Could you check a few things on this model? Use its own coordinates, in mm. Face numbers are marked on the shaded views. A direction names the side the tool comes from. Coordinates: 2 decimals unless noted, no trailing zeros. Loops run counter-clockwise (first coordinate to the right, second up) from the corner with the lowest first, then second, coordinate; pieces in that order, holes last. Notation, with made-up numbers: (5, 73) - (19, 73) arc R23 cw to (19, 99) - close; hole circle Ø5 at (-12.75, 46). An arc over 180 degrees is marked (long way). Put each result on its own line as item: value. Start each with the question number.
```python
from build123d import *

# Parameters (mm, degrees)
F0_R     = 3.175
F1_DEPTH = 12.7


with BuildPart() as f1:
    # F0 (on Front) → F1 (new body)
    with BuildSketch(Plane.XZ):
        with BuildLine():
            Line((0.507003, 7.684488), (0.507003, 6.329727))
            ThreePointArc((0.507003, 6.329727), (0, 6.35), (-0.507003, 6.329727))
            Line((-0.507003, 6.329727), (-0.507003, 7.684488))
            Line((-0.507003, 7.684488), (-0.257541, 7.684488))
            Line((-0.257541, 7.684488), (-0.257541, 7.937779))
            Line((-0.257541, 7.937779), (-0.507003, 7.937779))
            Line((-0.507003, 7.937779), (-1.277548, 7.937779))
            Line((-1.277548, 7.937779), (-1.277548, 6.220158))
            ThreePointArc((-1.277548, 6.220158), (-5.499261, 3.175), (-6.025589, -2.00369))
            Line((-6.025589, -2.00369), (-7.513093, -2.8625))
            Line((-7.513093, -2.8625), (-7.12782, -3.529812))
            Line((-7.12782, -3.529812), (-7.003089, -3.745852))
            Line((-7.003089, -3.745852), (-6.783733, -3.619207))
            Line((-6.783733, -3.619207), (-6.908463, -3.403167))
            Line((-6.908463, -3.403167), (-5.735206, -2.725786))
            ThreePointArc((-5.735206, -2.725786), (-5.499261, -3.175), (-5.228203, -3.603941))
            Line((-5.228203, -3.603941), (-6.401461, -4.281321))
            Line((-6.401461, -4.281321), (-6.526191, -4.065281))
            Line((-6.526191, -4.065281), (-6.745548, -4.191927))
            Line((-6.745548, -4.191927), (-6.620817, -4.407967))
            Line((-6.620817, -4.407967), (-6.235544, -5.075279))
            Line((-6.235544, -5.075279), (-4.748041, -4.216469))
            ThreePointArc((-4.748041, -4.216469), (0, -6.35), (4.748041, -4.216469))
            Line((4.748041, -4.216469), (6.235544, -5.075279))
            Line((6.235544, -5.075279), (6.620817, -4.407967))
            Line((6.620817, -4.407967), (6.745548, -4.191927))
            Line((6.745548, -4.191927), (6.526191, -4.065281))
            Line((6.526191, -4.065281), (6.401461, -4.281321))
            Line((6.401461, -4.281321), (5.228203, -3.603941))
            ThreePointArc((5.228203, -3.603941), (5.499261, -3.175), (5.735206, -2.725786))
            Line((5.735206, -2.725786), (6.908463, -3.403167))
            Line((6.908463, -3.403167), (6.783733, -3.619207))
            Line((6.783733, -3.619207), (7.003089, -3.745852))
            Line((7.003089, -3.745852), (7.12782, -3.529812))
            Line((7.12782, -3.529812), (7.513093, -2.8625))
            Line((7.513093, -2.8625), (6.025589, -2.00369))
            ThreePointArc((6.025589, -2.00369), (5.499261, 3.175), (1.277548, 6.220158))
            Line((1.277548, 6.220158), (1.277548, 7.937779))
            Line((1.277548, 7.937779), (0.507003, 7.937779))
            Line((0.507003, 7.937779), (0.257541, 7.937779))
            Line((0.257541, 7.937779), (0.257541, 7.684488))
            Line((0.257541, 7.684488), (0.507003, 7.684488))
        make_face()
        Circle(F0_R, mode=Mode.SUBTRACT)
    extrude(amount=F1_DEPTH)


solid = f1.part
```
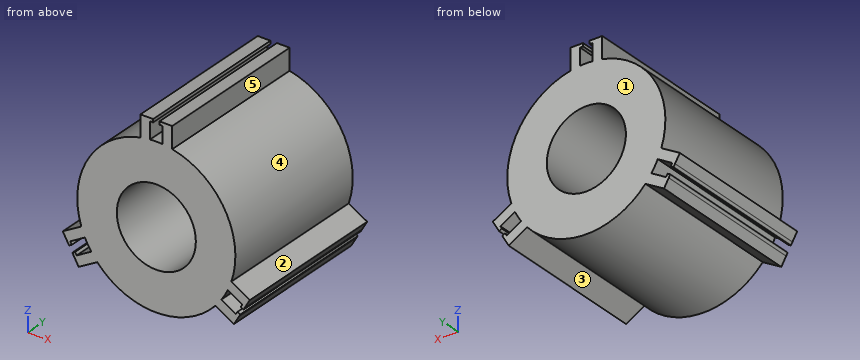
(1) Which directions (+Z, -Z, +X, -X, +Y, -Y) give clear straight access to the entire face, cutting with the end or side of a thin tool? Please do the marked faces 4 and 5.
(2) If we mould it in two halves opening along Z, with no side actions, what happens to the marked faces 1, 2 and 3? For each: pulls with the +Z half, pulls with the -Z half, needs draft (parallel to the pull), parting line crosses it, or undercut.
(3) For pin 1 Ø0.7 at (y, z) = (-5, 7) entering from -X; pin 2 Ø2 at (x, y) = (-2.5, -5) entering from +Z; pin 3 Ø0.5 at (y, z) = (-5.5, 7.5) entering from +X; pin 4 Ø5.5 at (x, z) = (0, 0) entering from +Y, each with a flat end and sliding along its axis, tell me the tip position at first contact or that it passes through.
(4) I want a section at C-C on z = 2.5. List the corners of the cut face in (x, y) for me.
(5) I want a section at B-B on x = -4.25. List the corners of the cut face in (y, z) for me, and give its area (3 significant figures).
(6) I want a section at D-D on z = 5. List the corners of the cut face in (x, y) for me.
(7) I want a section at A-A on z = 0. List the corners of the cut face in (x, y) for me (3 decimals).
(8) I need wall thicknesses on L1, parallel to Z at x = 0, y = -9.75 (3 decimals); L2, parallel to X at y = -7.5, z = -4.5; L3, parallel to X at y = -10.5, z = 7.25. Which ranges of each line are inside material? Lowest first, please. Write a range as [from, to].
Answer sheet:
1. face 4: +X, +Y, -Y
1. face 5: +Z, +X, +Y, -Y
2. face 1: needs draft
2. face 2: undercut
2. face 3: pulls with the -Z half
3. pin 1: stops at x = -1.28
3. pin 2: stops at z = 6.17
3. pin 3: stops at x = 1.28
3. pin 4: passes through
4. outline: (-5.84, -12.7) - (-1.96, -12.7) - (-1.96, 0) - (-5.84, 0) - close; (1.96, -12.7) - (5.84, -12.7) - (5.84, 0) - (1.96, 0) - close
5. outline: (-12.7, -4.72) - (0, -4.72) - (0, 4.72) - (-12.7, 4.72) - close
5. area: 120 mm^2
6. outline: (-3.91, -12.7) - (3.91, -12.7) - (3.91, 0) - (-3.91, 0) - close
7. outline: (-6.35, -12.7) - (-3.175, -12.7) - (-3.175, 0) - (-6.35, 0) - close; (3.175, -12.7) - (6.35, -12.7) - (6.35, 0) - (3.175, 0) - close
8. L1: z = [-6.35, -3.175], [3.175, 6.35]
8. L2: x = [-6.57, -5.24], [-4.48, 4.48], [5.24, 6.57]
8. L3: x = [-1.28, -0.51], [0.51, 1.28]
